Could you check a few things on this model? Use its own coordinates, in mm. Face numbers are marked on the shaded views. A direction names the side the tool comes from. Give positions to 0.01 mm unless a question says otherwise; leave off trailing zeros. Order: outer loops, then holes, each group sorted by start corner. A loop starts at its lowest first (then second) coordinate and runs counter-clockwise, first axis right, second up. Notation, with made-up numbers: (-9, 38.5) - (30, 38.5) arc R28 cw to (30, 60.5) - close; hole circle Ø10 at (89, 88.25). An arc over 180 degrees is marked (long way). Put each result on its own line as item: value.
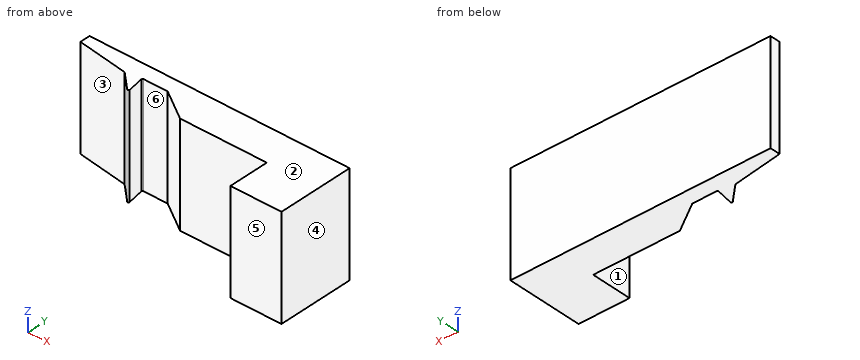
from build123d import *

# Parameters (mm, degrees)
BOSS_EXTRUDE1_DEPTH = 10
FILLET1_R           = 0.1


with BuildPart() as part:
    # Sketch1 → Boss-Extrude1 (new body)
    with BuildSketch(Plane.XY):
        Polygon((-17.64487365, -3.096839142), (-22.64487365, -3.096839142), (-22.64487365, 0.903160858), (-31.14487365, 0.903160858), (-34.14487365, 2.903160858), (-36.64487365, 2.903160858), (-36.294355732, 0.903160858), (-38.14487365, 2.653160858), (-43.14487365, 3.403160858), (-43.14487365, 4.403160858), (-17.64487365, 4.403160858), align=None)
    extrude(amount=BOSS_EXTRUDE1_DEPTH)

    # Fillet1
    fillet1_edges = [part.edges().sort_by_distance(p)[0] for p in [
        (-34.14487365, 2.903160858, 5),
        (-36.64487365, 2.903160858, 5),
        (-36.294355732, 0.903160858, 5),
    ]]
    fillet(fillet1_edges, radius=FILLET1_R)


solid = part.part
1) We'd pull the mould along X, two halves only. Please class the marked faces 3, 4, 5 and 6: pulls with the +X half, pulls with the -X half, needs draft (parallel to the pull), parting line crosses it, or undercut.
Filled in:
face 3: pulls with the -X half
face 4: pulls with the +X half
face 5: needs draft
face 6: undercut
2) If I drill on line 1 (Y direction, x = -24, z = 6.5); line 2 (X direction, y = -2.5, z = 8.5); line 3 (Y direction, x = -39, z = 5.75), over which ranges is the centre line in solid material (lowest first)? Write a range as [from, to].
Filled in:
line 1: y = [0.9, 4.4]
line 2: x = [-22.64, -17.64]
line 3: y = [2.78, 4.4]
3) Which directions (+Z, -Z, +X, -X, +Y, -Y) give clear straight access to the entire face, cutting with the end or side of a thin tool? Please do the marked faces 1 and 2.
Filled in:
face 1: +Z, -Z, -X, -Y
face 2: +Z, +X, -X, +Y, -Y
4) I'm going to push flat-ended pins straight in: pin 1 (4 mm diameter, centred on x = -28.5, z = 3.5, fed in from -Y); pin 2 (1.9 mm diameter, centred on x = -35, z = 6, fed in from -Y); pin 3 (1 mm diameter, centred on x = -39, z = 2.5, fed in from -Y). Where does each tip first touch, or does it pass through?
Filled in:
pin 1: stops at y = 0.9
pin 2: stops at y = 2.84
pin 3: stops at y = 2.71
5) Suppose I cut it at A-A, the plane z = 5.5. List the corners of the cut face in (x, y) for me.
Filled in:
outline: (-43.14, 3.4) - (-38.14, 2.65) - (-36.51, 1.11) arc R0.1 ccw to (-36.35, 1.2) - (-36.62, 2.79) arc R0.1 cw to (-36.53, 2.9) - (-34.18, 2.9) arc R0.1 cw to (-34.12, 2.89) - (-31.14, 0.9) - (-22.64, 0.9) - (-22.64, -3.1) - (-17.64, -3.1) - (-17.64, 4.4) - (-43.14, 4.4) - close
6) Suppose I cut it at C-C, the plane y = 0.25. List the corners of the cut face in (x, z) for me, and give its area (3 significant figures).
Filled in:
outline: (-22.64, 0) - (-17.64, 0) - (-17.64, 10) - (-22.64, 10) - close
area: 50.0 mm^2
7) Suppose I cut it at B-B, the plane x = -34.5. List the corners of the cut face in (y, z) for me, and give its area (3 significant figures).
Filled in:
outline: (2.9, 0) - (4.4, 0) - (4.4, 10) - (2.9, 10) - close
area: 15.0 mm^2
